```python
from build123d import *

# Parameters (mm, degrees)
F0_R     = 15
F0_R_2   = 11.2
F1_DEPTH = 3.5
F2_R     = 15
F3_DEPTH = 0.4
F4_R     = 4.2
F5_DEPTH = 7.801


# Not quite as in the source:
# - a pattern or mirror of a feature is missing from the dataset's text; its kind, count and spacing are read off the source's solid


with BuildPart() as f1:
    # F0 (on Top) → F1 (new body, symmetric)
    with BuildSketch(Plane.XY):
        Circle(F0_R)
        Circle(F0_R_2, mode=Mode.SUBTRACT)
    extrude(amount=F1_DEPTH, both=True)

    # F2 (on face) → F3 (join)
    with BuildSketch(Plane(origin=(0, 0, -3.5), x_dir=(1, 0, 0), z_dir=(0, 0, -1))):
        Circle(F2_R)
    f3 = extrude(amount=F3_DEPTH)

    # F3_copies: F3 across plane
    add(f3.mirror(Plane.XY))

    # F4 (on face) → F5 (cut, through all)
    with BuildSketch(Plane(origin=(0, 0, -3.9), x_dir=(1, 0, 0), z_dir=(0, 0, -1))):
        Circle(F4_R)
    extrude(amount=-F5_DEPTH, mode=Mode.SUBTRACT)


solid = f1.part
```
Input: part model. Units: mm. Frame: model coordinates. A direction names the side the tool comes from. Coordinates: 2 decimals unless noted, no trailing zeros. Write each loop counter-clockwise with the first axis right and the second up, starting at its lowest first coordinate (ties: lowest second). Pieces come first, ordered by that corner, then holes.
1) Section D-D on y = 6.5. Output: boundary loops of the cut face in (x, z).
2) Mould query, pull axis Z, two halves, no side actions, for faces 3 (the flat face through (0, 5, -3.5)), 4 (the cylindrical face through (4.006, -1.262, -3.703)), 5 (the cylindrical face through (-11.19, 0.49, -0.05)), 6 (the flat face through (3.1, 3.1, 3.9)). Classes: pulls with the +Z half, pulls with the -Z half, needs draft (parallel to the pull), parting line crosses it, or undercut.
3) Pin query (flat end, axial travel): pin 1 Ø5 at (x, y) = (0, 0) entering from +Z; pin 2 Ø3 at (y, z) = (9, 1) entering from +X; pin 3 Ø3 at (y, z) = (-8, 2.5) entering from -X. Return the tip coordinate at first contact, or that it passes through.
4) Material intervals for line 1 along Y through (x, z) = (0, -3.7); line 2 along Z through (x, y) = (-0.75, 5.75), sorted ascending.
5) Section A-A on y = 0. Output: boundary loops of the cut face in (x, z).
6) Set-up query: faces 1 (the flat face through (0, 5, 3.5)), 2 (the flat face through (3.1, 3.1, -3.9)). Return all of +Z, -Z, +X, -X, +Y, -Y with unobstructed straight access to the full face (end or side cutting, diameter ignored); none if empty.
7) Section C-C on x = -6.25. Output: boundary loops of the cut face in (y, z), and give its area (3 significant figures).
Check result:
1. outline: (-13.52, -3.9) - (13.52, -3.9) - (13.52, 3.9) - (-13.52, 3.9) - close; hole (-9.12, -3.5) - (9.12, -3.5) - (9.12, 3.5) - (-9.12, 3.5) - close
2. face 3: undercut
2. face 4: needs draft
2. face 5: undercut
2. face 6: pulls with the +Z half
3. pin 1: passes through
3. pin 2: stops at x = 12.99
3. pin 3: stops at x = -13.52
4. line 1: y = -15 to -4.2, 4.2 to 15
4. line 2: z = -3.9 to -3.5, 3.5 to 3.9
5. outline: (-15, -3.9) - (-4.2, -3.9) - (-4.2, -3.5) - (-11.2, -3.5) - (-11.2, 3.5) - (-4.2, 3.5) - (-4.2, 3.9) - (-15, 3.9) - close; (4.2, -3.9) - (15, -3.9) - (15, 3.9) - (4.2, 3.9) - (4.2, 3.5) - (11.2, 3.5) - (11.2, -3.5) - (4.2, -3.5) - close
6. face 1: none
6. face 2: -Z, +X, -X, +Y, -Y
7. outline: (-13.64, -3.9) - (13.64, -3.9) - (13.64, 3.9) - (-13.64, 3.9) - close; hole (-9.29, -3.5) - (9.29, -3.5) - (9.29, 3.5) - (-9.29, 3.5) - close
7. area: 82.6 mm2
